Model file for the job. Use its own axes, mm. Face numbers are marked on the shaded views. Give positions to 0.01 mm unless a question says otherwise; leave off trailing zeros. Write each loop counter-clockwise with the first axis right and the second up, starting at its lowest first coordinate (ties: lowest second). Pieces come first, ordered by that corner, then holes. Notation, with made-up numbers: (45.25, 44.5) - (100.25, 44.5) arc R20 ccw to (100.25, 64.5) - close; hole circle Ø6 at (7, -11). An arc over 180 degrees is marked (long way). Use CSV: the item, a comma, the result in double quotes.
from build123d import *

# Parameters (mm, degrees)
SKETCH2_R           = 1.625
BOSS_EXTRUDE1_DEPTH = 4
FILLET1_R           = 3


with BuildPart() as part:
    # Sketch2 → Boss-Extrude1 (new body)
    with BuildSketch(Plane.XY):
        Polygon((0, 0), (20, 0), (20, 7.5), (-20, 7.5), (-20, 0), align=None)
        with Locations((16.25, 3.75)):
            Circle(SKETCH2_R, mode=Mode.SUBTRACT)
        with Locations(Location((-16.25, 3.75, 0), (0, 0, 180))):
            Circle(SKETCH2_R, mode=Mode.SUBTRACT)
    extrude(amount=BOSS_EXTRUDE1_DEPTH)

    # Fillet1
    fillet1_edges = [part.edges().sort_by_distance(p)[0] for p in [
        (-20, 0, 2),
        (-20, 7.5, 2),
        (20, 7.5, 2),
        (20, 0, 2),
    ]]
    fillet(fillet1_edges, radius=FILLET1_R)


solid = part.part
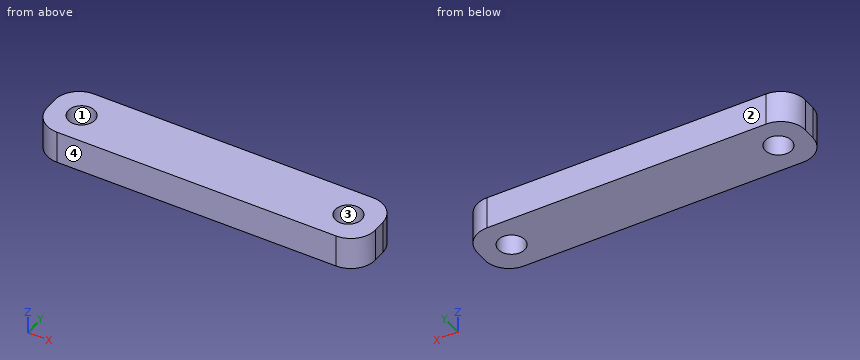
(1) Saw through at C-C, the plane z = 2.3. List the corners of the cut face in (x, y) (3 decimals), then the cut area to 3 significant figures.
Checked values:
outline,"(-20, 3) arc R3 ccw to (-17, 0) - (17, 0) arc R3 ccw to (20, 3) - (20, 4.5) arc R3 ccw to (17, 7.5) - (-17, 7.5) arc R3 ccw to (-20, 4.5) - close; hole circle Ø3.25 at (-16.25, 3.75); hole circle Ø3.25 at (16.25, 3.75)"
area,"276 mm^2"
(2) Saw through at D-D, the plane y = 7. List the corners of the cut face in (x, z).
Checked values:
outline,"(-18.66, 0) - (18.66, 0) - (18.66, 4) - (-18.66, 4) - close"
(3) Wall check: probe 1 along Y at (x, z) = (-16.25, 1.05) (3 decimals); probe 2 along X at (y, z) = (2.5, 2.9); probe 3 along X at (y, z) = (5.5, 3.25). Give the ranges that are in metal, low to high. Write a range as [from, to].
Checked values:
probe 1,"y = [0, 2.125], [5.375, 7.5]"
probe 2,"x = [-19.96, -17.29], [-15.21, 15.21], [17.29, 19.96]"
probe 3,"x = [-19.83, 19.83]"
(4) Pull direction Y, two halves, no side cores. Call the marked faces 1, 2, 3 and 4: released by +Y, released by -Y, zero draft, split by the parting line, or undercut.
Checked values:
face 1,"undercut"
face 2,"released by +Y"
face 3,"undercut"
face 4,"released by -Y"
(5) Saw through at A-A, the plane x = 16.25. List the corners of the cut face in (y, z) (3 decimals), then the cut area to 3 significant figures.
Checked values:
outline,"(0, 0) - (2.125, 0) - (2.125, 4) - (0, 4) - close; (5.375, 0) - (7.5, 0) - (7.5, 4) - (5.375, 4) - close"
area,"17.0 mm^2"
(6) Saw through at B-B, the plane y = 3.75. List the corners of the cut face in (x, z) (3 decimals), then the cut area to 3 significant figures.
Checked values:
outline,"(-20, 0) - (-17.875, 0) - (-17.875, 4) - (-20, 4) - close; (-14.625, 0) - (14.625, 0) - (14.625, 4) - (-14.625, 4) - close; (17.875, 0) - (20, 0) - (20, 4) - (17.875, 4) - close"
area,"134 mm^2"
